Could you check a few things on this model? Use its own coordinates, in mm. A direction names the side the tool comes from. Coordinates: 2 decimals unless noted, no trailing zeros. Loops run counter-clockwise (first coordinate to the right, second up) from the corner with the lowest first, then second, coordinate; pieces in that order, holes last. Notation, with made-up numbers: M -31,78.5 L 10,78.5 A33 ccw 10,107.5 Z; hole C -7,4.5 d10. An arc over 180 degrees is marked long. Write each question's results on one line, items separated by ' | '.
```python
from build123d import *

# Parameters (mm, degrees)
SKETCH2_R           = 4.5
BOSS_EXTRUDE1_DEPTH = 12
SKETCH4_R           = 5.5
SKETCH4_R_2         = 4.5
BOSS_EXTRUDE3_DEPTH = 1


with BuildPart() as part:
    # Sketch2 → Boss-Extrude1 (new body)
    with BuildSketch(Plane(origin=(0, 0, 0), x_dir=(1, 0, 0), z_dir=(0, 1, 0))):
        Circle(SKETCH2_R)
        Polygon((4.041451884, 0), (2.020725942, 3.5), (-2.020725942, 3.5), (-4.041451884, 0), (-2.020725942, -3.5), (2.020725942, -3.5), align=None, mode=Mode.SUBTRACT)
    extrude(amount=BOSS_EXTRUDE1_DEPTH)

    # Sketch4 → Boss-Extrude3 (add)
    with BuildSketch(Plane.XZ):
        Circle(SKETCH4_R)
        Circle(SKETCH4_R_2, mode=Mode.SUBTRACT)
    extrude(amount=-BOSS_EXTRUDE3_DEPTH)


solid = part.part
```
(1) Imagine slicing it at D-D, the plane x = -4.25. List the corners of the cut face in (y, z) for me.
Reported:
outline: M 0,-3.49 L 1,-3.49 L 1,-1.48 L 12,-1.48 L 12,1.48 L 1,1.48 L 1,3.49 L 0,3.49 Z
(2) If we mould it in two halves opening along Z, with no side actions, what happens to faces 1 (the flat face through (3, 5.9, 1.8)), 2 (the cylindrical face through (-1.19, 0.49, -5.37)), 3 (the flat face through (0, 12, -4))? For each: released by +Z, released by -Z, zero draft, split by the parting line, or undercut.
Reported:
face 1: undercut | face 2: split by the parting line | face 3: zero draft
(3) Imagine slicing it at B-B, the plane x = 0. List the corners of the cut face in (y, z) for me.
Reported:
outline: M 0,-5.5 L 1,-5.5 L 1,-4.5 L 12,-4.5 L 12,-3.5 L 0,-3.5 Z; M 0,3.5 L 12,3.5 L 12,4.5 L 1,4.5 L 1,5.5 L 0,5.5 Z
(4) Will these pins go through, and if not, where does the flat tip stop? P1, Ø2, axis at x = -0.5, y = 7.5, coming from the -Z side; P2, Ø2, axis at x = 0, y = 5.5, coming from the +Z side.
Reported:
P1: stops at z = -4.5 | P2: stops at z = 4.5
(5) Imagine slicing it at A-A, the plane y = 6. List the corners of the cut face in (x, z) for me.
Reported:
outline: C 0,0 d9; hole M -4.04,0 L -2.02,-3.5 L 2.02,-3.5 L 4.04,0 L 2.02,3.5 L -2.02,3.5 Z
(6) Which directions (+Z, -Z, +X, -X, +Y, -Y) give clear straight access to the entire face, cutting with the end or side of a thin tool? Please do faces 4 (the flat face through (0, 0, -4)), 5 (the flat face through (-5, 1, 0)), 6 (the flat face through (3.045, 5.916, -1.726)).
Reported:
face 4: +Z, -Z, +X, -X, -Y | face 5: +Y | face 6: +Y, -Y
(7) Imagine slicing it at C-C, the plane z = 2.75. List the corners of the cut face in (x, y) for me, and give its area (3 significant figures).
Reported:
outline: M -4.76,0 L -2.45,0 L -2.45,12 L -3.56,12 L -3.56,1 L -4.76,1 Z; M 2.45,0 L 4.76,0 L 4.76,1 L 3.56,1 L 3.56,12 L 2.45,12 Z | area: 29.0 mm2
(8) Please list where these lines run through material, in increasing order: probe 1 along Z at (x, y) = (-3.75, 6); probe 2 along X at (y, z) = (9.5, -2); probe 3 along X at (y, z) = (4.75, -1.5). Write a range as from..to.
Reported:
probe 1: z = -2.49..-0.5, 0.5..2.49 | probe 2: x = -4.03..-2.89, 2.89..4.03 | probe 3: x = -4.24..-3.18, 3.18..4.24
